```python
from build123d import *

# Parameters (mm, degrees)
F1_DEPTH = 10
F2_R     = 10
F3_DEPTH = 25
F4_R     = 5
F5_DEPTH = 25


with BuildPart() as f1:
    # F0 (on Front) → F1 (new body)
    with BuildSketch(Plane.XZ):
        with BuildLine():
            ThreePointArc((4.7458544305, 33.6244736514), (2.4011029044, 34.1735286962), (0, 34.3579900832))
            ThreePointArc((0, 34.3579900832), (-2.4011029044, 34.1735286962), (-4.7458544305, 33.6244736514))
            add(Edge.make_bspline(
                [(-4.7458544305, 33.6244736514), (-10.9520952223, 31.6590568221), (-16.416283898, 13.4392161658), (-27.7037138128, 8.8834728939), (-30.1568813613, 0)],
                knots=[0, 0, 0, 0, 0.5039121185, 1, 1, 1, 1], degree=3))
            ThreePointArc((-30.1568813613, 0), (-24.893077801, -27.2783942003), (0, -39.6134294928))
            ThreePointArc((0, -39.6134294928), (24.893077801, -27.2783942003), (30.1568813613, 0))
            add(Edge.make_bspline(
                [(4.7458544305, 33.6244736514), (10.9520952223, 31.6590568221), (16.416283898, 13.4392161658), (27.7037138128, 8.8834728939), (30.1568813613, 0)],
                knots=[0, 0, 0, 0, 0.5039121185, 1, 1, 1, 1], degree=3))
        make_face()
    extrude(amount=F1_DEPTH)

    # F2 (on face) → F3 (cut)
    with BuildSketch(Plane.XZ.offset(10)):
        with Locations((0, -20)):
            Circle(F2_R)
    extrude(amount=-F3_DEPTH, mode=Mode.SUBTRACT)

    # F4 (on face) → F5 (cut)
    with BuildSketch(Plane.XZ.offset(10)):
        with Locations((0, 19.0365062821)):
            Circle(F4_R)
    extrude(amount=-F5_DEPTH, mode=Mode.SUBTRACT)


solid = f1.part
```
Geometry: final body of the model. Coordinates: model frame, mm. Coordinates: 2 decimals unless noted, no trailing zeros. Order: outer loops, then holes, each group sorted by start corner. A loop starts at its lowest first (then second) coordinate and runs counter-clockwise, first axis right, second up. Notation, with made-up numbers: M -22.75,1.25 L 8.25,1.25 A20 ccw 8.25,38.25 Z; hole C -11,13 d5. An arc over 180 degrees is marked long. Answer in a Markdown table with one row per item. Add a question column.
Q1. Mould query, pull axis Z, two halves, no side actions, for faces 1 (the cylindrical face through (-1.302, -5.07, -10.085)), 2 (the flat face through (0, 0, -2)), 3 (the cylindrical face through (-0.806, -4.93, -39.603)). Classes: released by +Z, released by -Z, zero draft, split by the parting line, or undercut.
Q2. Contact query for flat-ended pins moving along their axis: P1, Ø1.5, axis at y = -1.5, z = 25, coming from the +X side; P2, Ø3, axis at y = -7.5, z = 14.5, coming from the -X side; P3, Ø1.5, axis at y = -8.5, z = 0.5, coming from the -X side. Output: stop coordinate, or through.
Q3. Section query A-A on z = -24. Return the cut outline in (x, y).
Q4. Line query: L1, parallel to Z at x = 0, y = -5; L2, parallel to Z at x = -6, y = -9; L3, parallel to X at y = -9.25, z = -29. Output: solid intervals per line, ascending.
Q5. Section query B-B on y = -4.5. Count the separate pieces of the cut face and the enclosed holes in it, and give its area (3 significant figures).
Completed:
| question | item | result |
|---|---|---|
| 1 | face 1 | undercut |
| 1 | face 2 | zero draft |
| 1 | face 3 | split by the parting line |
| 2 | P1 | stops at x = 13.45 |
| 2 | P2 | stops at x = -21.28 |
| 2 | P3 | stops at x = -30.22 |
| 3 | outline | M -27.08,-10 L -9.17,-10 L -9.17,0 L -27.08,0 Z; M 9.17,-10 L 27.08,-10 L 27.08,0 L 9.17,0 Z |
| 4 | L1 | z = -39.61 to -30, -10 to 14.04, 24.04 to 34.36 |
| 4 | L2 | z = -39.03 to -28, -12 to 33.11 |
| 4 | L3 | x = -23.48 to -4.36, 4.36 to 23.48 |
| 5 | separate pieces | 1 |
| 5 | enclosed holes | 2 |
| 5 | area | 2,930 mm2 |
